The figure shows three views and two pictorial views of one solid part (mm, origin at its lowest corner). Answer the questions. A direction names the side the tool comes from. Coordinates: 2 decimals unless noted, no trailing zeros. Loops run counter-clockwise (first coordinate to the right, second up) from the corner with the lowest first, then second, coordinate; pieces in that order, holes last. Notation, with made-up numbers: (24.25, 77.25) -> (77.25, 77.25) arc R23 ccw to (77.25, 97.25) -> close; hole circle Ø11 at (51, -17.75). An arc over 180 degrees is marked (long way). Answer in a Markdown table with one row per item.
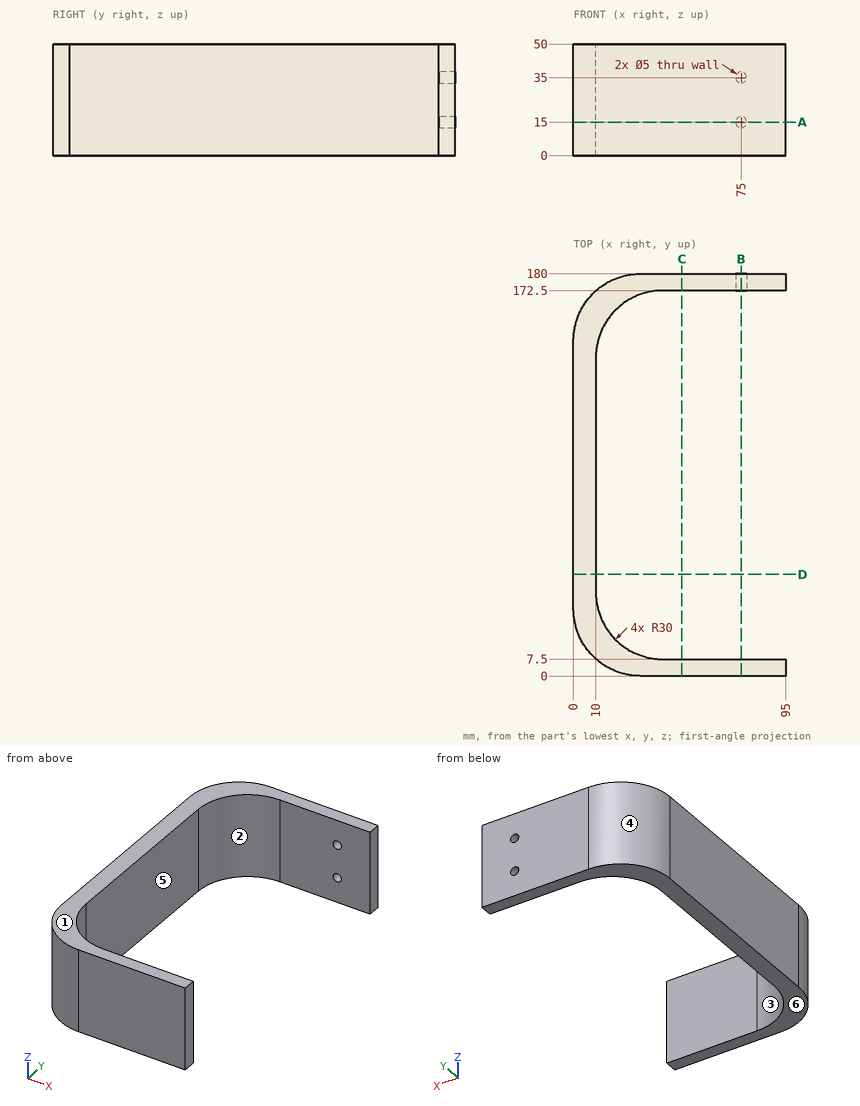
Item 1: A cutting plane is placed at D-D, the plane y = 45.5. Determine the outline of the cut face in (x, z), plus the area to 3 significant figures.
Findings below:
| item | result |
|---|---|
| outline | (0, 0) -> (10, 0) -> (10, 50) -> (0, 50) -> close |
| area | 500 mm2 |
Item 2: Find the intervals of material crossed by probe 1 along Y at (x, z) = (61.5, 18.5); probe 2 along X at (y, z) = (177.25, 15); probe 3 along X at (y, z) = (129, 13), in increasing order.
Findings below:
| item | result |
|---|---|
| probe 1 | y = 0 to 7.5, 172.5 to 180 |
| probe 2 | x = 17.45 to 72.5, 77.5 to 95 |
| probe 3 | x = 0 to 10 |
Item 3: A cutting plane is placed at A-A, the plane z = 15. Determine the outline of the cut face in (x, y).
Findings below:
| item | result |
|---|---|
| outline | (0, 30) arc R30 ccw to (30, 0) -> (95, 0) -> (95, 7.5) -> (40, 7.5) arc R30 cw to (10, 37.5) -> (10, 142.5) arc R30 cw to (40, 172.5) -> (72.5, 172.5) -> (72.5, 180) -> (30, 180) arc R30 ccw to (0, 150) -> close; (77.5, 172.5) -> (95, 172.5) -> (95, 180) -> (77.5, 180) -> close |
Item 4: A tool of negligible diameter and unlimited length cuts with its end or side. For the marked faces 1 and 2, from which of +Z, -Z, +X, -X, +Y, -Y can it reach the whole face along a straight path? Write none if from no direction.
Findings below:
| item | result |
|---|---|
| face 1 | +Z, +X, -X, +Y, -Y |
| face 2 | +Z, -Z, +X |
Item 5: A cutting plane is placed at B-B, the plane x = 75. Determine the outline of the cut face in (y, z), plus the area to 3 significant figures.
Findings below:
| item | result |
|---|---|
| outline | (0, 0) -> (7.5, 0) -> (7.5, 50) -> (0, 50) -> close; (172.5, 0) -> (180, 0) -> (180, 12.5) -> (172.5, 12.5) -> close; (172.5, 17.5) -> (180, 17.5) -> (180, 32.5) -> (172.5, 32.5) -> close; (172.5, 37.5) -> (180, 37.5) -> (180, 50) -> (172.5, 50) -> close |
| area | 675 mm2 |
Item 6: Determine the mould class of the marked faces 3, 4, 5 and 6 for opening direction Y: +Y half, -Y half, draft (parallel to the pull), parting line (faces both ways), or undercut.
Findings below:
| item | result |
|---|---|
| face 3 | undercut |
| face 4 | +Y half |
| face 5 | undercut |
| face 6 | draft |
Item 7: A cutting plane is placed at C-C, the plane x = 48.5. Determine the outline of the cut face in (y, z).
Findings below:
| item | result |
|---|---|
| outline | (0, 0) -> (7.5, 0) -> (7.5, 50) -> (0, 50) -> close; (172.5, 0) -> (180, 0) -> (180, 50) -> (172.5, 50) -> close |
Item 8: A flat-ended cylindrical pin translates along its axis: pin 1 Ø4 at (x, z) = (75, 15) entering from +Y. Find the tip coordinate at first contact, or state that the pin passes through.
Findings below:
| item | result |
|---|---|
| pin 1 | stops at y = 7.5 |
